```python
from build123d import *

# Parameters (mm, degrees)
SKETCH002_W                                = 12
SKETCH002_H                                = 13
SKETCH002_R                                = 0.95
PAD001007_DEPTH                            = 2
SKETCH003_W                                = 2
SKETCH003_H                                = 13
PAD002_DEPTH                               = 5.75
SKETCH004_R                                = 2.6
POCKET001_DEPTH                            = 1
CHAMFER005021077002006007019003032014_SIZE = 1
CHAMFER001_SIZE                            = 1
CHAMFER002_SIZE                            = 0.4


with BuildPart() as part:
    # Sketch002 → Pad001007 (new body)
    with BuildSketch(Plane.XY):
        with Locations((6, 0)):
            Rectangle(SKETCH002_W, SKETCH002_H)
        with Locations((6.75, 3.25)):
            Circle(SKETCH002_R, mode=Mode.SUBTRACT)
        with Locations((6.75, -3.25)):
            Circle(SKETCH002_R, mode=Mode.SUBTRACT)
    extrude(amount=PAD001007_DEPTH)

    # Sketch003 (on Face8 of Pad001007) → Pad002 (join)
    with BuildSketch(Plane.XY.offset(2)):
        with Locations((1, 0)):
            Rectangle(SKETCH003_W, SKETCH003_H)
    extrude(amount=PAD002_DEPTH)

    # Sketch004 (on Face4 of Pad002) → Pocket001 (cut)
    with BuildSketch(Plane(origin=(0, 0, 0), x_dir=(1, 0, 0), z_dir=(0, 0, -1))):
        with Locations((6.75, 3.25)):
            Circle(SKETCH004_R)
        with Locations((6.75, -3.25)):
            Circle(SKETCH004_R)
    extrude(amount=-POCKET001_DEPTH, mode=Mode.SUBTRACT)

    # Chamfer005021077002006007019003032014
    chamfer005021077002006007019003032014_edges = [part.edges().sort_by_distance(p)[0] for p in [
        (0, 0, 0),
    ]]
    chamfer(chamfer005021077002006007019003032014_edges, length=CHAMFER005021077002006007019003032014_SIZE)

    # Chamfer001
    chamfer001_edges = [part.edges().sort_by_distance(p)[0] for p in [
        (2, 6.5, 4.875),
        (2, -6.5, 4.875),
    ]]
    chamfer(chamfer001_edges, length=CHAMFER001_SIZE)

    # Chamfer002
    chamfer002_edges = [part.edges().sort_by_distance(p)[0] for p in [
        (12, 6.5, 1),
        (12, -6.5, 1),
    ]]
    chamfer(chamfer002_edges, length=CHAMFER002_SIZE)


solid = part.part
```
Design review of the part built by this model. Coordinates are the model's own, in mm. A direction names the side the tool comes from. Round coordinates to 2 decimals unless told otherwise and drop trailing zeros. Write each loop counter-clockwise with the first axis right and the second up, starting at its lowest first coordinate (ties: lowest second). Pieces come first, ordered by that corner, then holes.
Item 1: The part is to be moulded in two halves that separate along X. For faces 1 (the flat face through (2, 0, 5)), 2 (the flat face through (1, 0, 7.75)), 3 (the cylindrical face through (5.8, 3.3, 1.5)), 4 (the flat face through (0.5, -0.1, 0.5)), say which applies: +X half, -X half, draft (parallel to the pull), parting line (faces both ways), or undercut.
Item 2: We need section D-D on y = 0. Write out the cut boundary in (x, z).
Item 3: We need section B-B on z = 1.75. Write out the cut boundary in (x, y), and give its area (3 significant figures).
Item 4: For probe 1 along Y at (x, z) = (6.75, 0.5); probe 2 along Y at (x, z) = (6.75, 1.6); probe 3 along X at (y, z) = (-3.25, 1.6), list the stretches that pass through material, from the lowest coordinate up.
Item 5: We need section A-A on y = -3.25. Write out the cut boundary in (x, z).
Item 6: We need section C-C on x = 8. Write out the cut boundary in (y, z).
Item 7: For faces 5 (the cylindrical face through (7.95, -0.943, 0.493)), 6 (the flat face through (1.5, 6, 4.8)), 7 (the flat face through (1.5, -6, 4.8)), 8 (the flat face through (4.9, 6.5, 1.8)), 9 (the flat face through (12, 0, 1)), list the 3-axis set-ups (+Z, -Z, +X, -X, +Y, -Y) from which the entire face can be reached by the end or side of a thin tool; tool diameter is ignored.
Item 8: Clearance check with flat-ended pins moving along their axes: pin 1 Ø2.5 at (x, y) = (6.75, 3.25) entering from -Z; pin 2 Ø4.5 at (y, z) = (-1, 5) entering from +X; pin 3 Ø1.5 at (x, y) = (5.5, -0.5) entering from +Z; pin 4 Ø1.7 at (x, y) = (6.75, -3.25) entering from -Z. State where each tip first meets the part, or that it passes through.
Returned:
1. face 1: +X half
1. face 2: draft
1. face 3: undercut
1. face 4: -X half
2. outline: (0, 1) - (1, 0) - (12, 0) - (12, 2) - (2, 2) - (2, 7.75) - (0, 7.75) - close
3. outline: (0, -6.5) - (11.6, -6.5) - (12, -6.1) - (12, 6.1) - (11.6, 6.5) - (0, 6.5) - close; hole circle Ø1.9 at (6.75, -3.25); hole circle Ø1.9 at (6.75, 3.25)
3. area: 150 mm2
4. probe 1: y = -6.5 to -5.85, -0.65 to 0.65, 5.85 to 6.5
4. probe 2: y = -6.5 to -4.2, -2.3 to 2.3, 4.2 to 6.5
4. probe 3: x = 0 to 5.8, 7.7 to 12
5. outline: (0, 1) - (1, 0) - (4.15, 0) - (4.15, 1) - (5.8, 1) - (5.8, 2) - (2, 2) - (2, 7.75) - (0, 7.75) - close; (7.7, 1) - (9.35, 1) - (9.35, 0) - (12, 0) - (12, 2) - (7.7, 2) - close
6. outline: (-6.5, 0) - (-5.53, 0) - (-5.53, 1) - (-0.97, 1) - (-0.97, 0) - (0.97, 0) - (0.97, 1) - (5.53, 1) - (5.53, 0) - (6.5, 0) - (6.5, 2) - (-6.5, 2) - close
7. face 5: -Z
7. face 6: +Z, +X, +Y
7. face 7: +Z, +X, -Y
7. face 8: +Z, -Z, +X, -X, +Y
7. face 9: +Z, -Z, +X, +Y, -Y
8. pin 1: stops at z = 1
8. pin 2: stops at x = 2
8. pin 3: stops at z = 2
8. pin 4: passes through
